Part print with two shaded views. Sizes in mm from the minimum x, y, z corner. A direction names the side the tool comes from. Coordinates: 2 decimals unless noted, no trailing zeros. Loops run counter-clockwise (first coordinate to the right, second up) from the corner with the lowest first, then second, coordinate; pieces in that order, holes last. Notation, with made-up numbers: (4, -34.5) -> (57, -34.5) arc R14 cw to (57, -11.5) -> close; hole circle Ø2 at (16.25, 28.5). An arc over 180 degrees is marked (long way). Use one line per item in the form item = value.
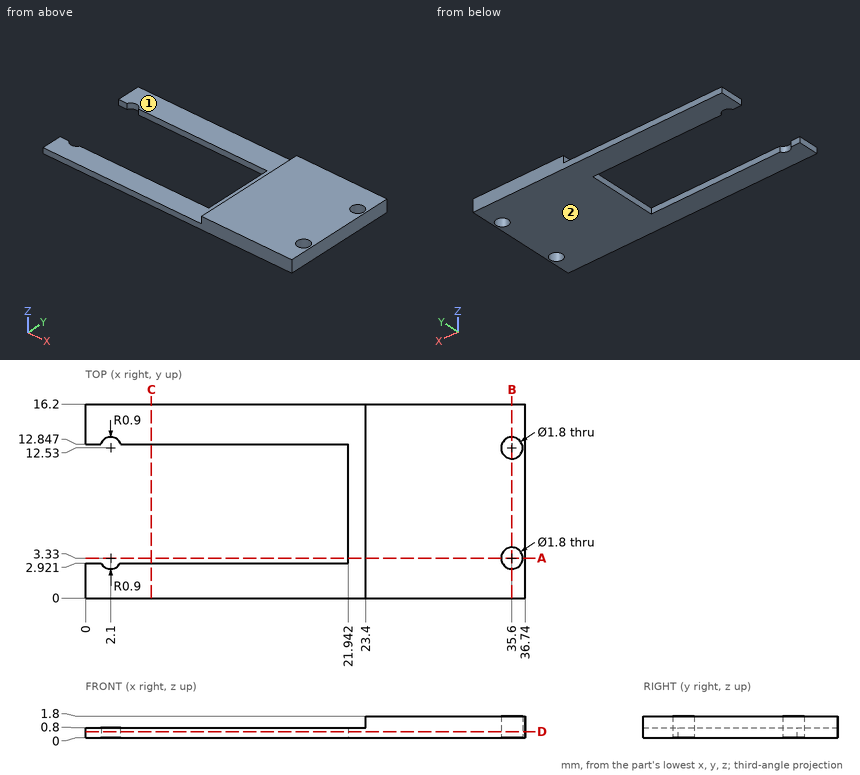
Q1. Band-saw the part on B-B, the plane x = 35.6. Write the cut outline in (y, z), and give its area (3 significant figures).
Result:
outline = (0, 0) -> (2.43, 0) -> (2.43, 1.8) -> (0, 1.8) -> close; (4.23, 0) -> (11.63, 0) -> (11.63, 1.8) -> (4.23, 1.8) -> close; (13.43, 0) -> (16.2, 0) -> (16.2, 1.8) -> (13.43, 1.8) -> close
area = 22.7 mm2
Q2. Band-saw the part on A-A, the plane y = 3.33. Write the cut outline in (x, z).
Result:
outline = (21.94, 0) -> (34.7, 0) -> (34.7, 1.8) -> (23.4, 1.8) -> (23.4, 0.8) -> (21.94, 0.8) -> close; (36.5, 0) -> (36.74, 0) -> (36.74, 1.8) -> (36.5, 1.8) -> close
Q3. Pin check, flat tips, straight feed: pin 1 Ø0.8 at (y, z) = (6.5, 1.5) entering from -X; pin 2 Ø0.9 at (y, z) = (6, 0.5) entering from -X. Stop position of each tip, or through.
Result:
pin_1 = 23.4
pin_2 = 21.94
Q4. Which spindle directions (+Z, -Z, +X, -X, +Y, -Y) get a long thin tool onto all of the face, cutting with end or side? Do the marked faces 1 and 2. Say none if no direction does.
Result:
face_1 = +Z, -X, +Y, -Y
face_2 = -Z, +X, -X, +Y, -Y
Q5. Band-saw the part on C-C, the plane x = 5.5. Write the cut outline in (y, z).
Result:
outline = (0, 0) -> (2.92, 0) -> (2.92, 0.8) -> (0, 0.8) -> close; (12.85, 0) -> (16.2, 0) -> (16.2, 0.8) -> (12.85, 0.8) -> close
Q6. Band-saw the part on D-D, the plane z = 0.5. Write the cut outline in (x, y), and give its area (3 significant figures).
Result:
outline = (0, 0) -> (36.74, 0) -> (36.74, 16.2) -> (0, 16.2) -> (0, 12.85) -> (1.26, 12.85) arc R0.9 cw to (2.94, 12.85) -> (21.94, 12.85) -> (21.94, 2.92) -> (2.9, 2.92) arc R0.9 cw to (1.3, 2.92) -> (0, 2.92) -> close; hole circle Ø1.8 at (35.6, 3.33); hole circle Ø1.8 at (35.6, 12.53)
area = 371 mm2
Q7. Wall check: line 1 along Y through (x, z) = (35.6, 1.3); line 2 along Y through (x, z) = (3.5, 0.1); line 3 along X through (y, z) = (7.25, 0.85). Give the ranges that are in metal, low to high.
Result:
line_1 = 0 to 2.43, 4.23 to 11.63, 13.43 to 16.2
line_2 = 0 to 2.92, 12.85 to 16.2
line_3 = 23.4 to 36.74
